Geometry check sheet. Reference: the model listing, model coordinates, mm. A direction names the side the tool comes from. Give positions to 0.01 mm unless a question says otherwise; leave off trailing zeros. Write each loop counter-clockwise with the first axis right and the second up, starting at its lowest first coordinate (ties: lowest second). Pieces come first, ordered by that corner, then holes.
(1) Depth check by flat-ended pin: P1, Ø12, axis at x = -33, z = 26.5, coming from the -Y side; P2, Ø4.5, axis at x = 50, y = -25, coming from the +Z side. Enter the tip coordinate at first touch or a pass-through.
(2) Cross-section at A-A (y = -31.5). Record the boundary of the cut face in (x, z).
(3) Thickness scan on line 1 along X through (y, z) = (-25, -96.25); line 2 along Z through (x, y) = (10, -27); line 3 along Y through (x, z) = (-50, -96). Record the ranges inside material, lowest first.
(4) Mould release check, pull along Z, two halves, no side actions. Record for faces 3 (the flat face through (-2, -22, -100)), 4 (the flat face through (-12, -45, -96)), 5 (the flat face through (-2, -30, 90)), 6 (the flat face through (-2, -15, 1)): +Z half, -Z half, draft (parallel to the pull), parting line (faces both ways), or undercut.
(5) Cross-section at B-B (x = -65). Record the boundary of the cut face in (y, z).
(6) Tool access check on faces 1 (the flat face through (-150, -22, -1)), 2 (the flat face through (-140, -30, -1)). Record the directions out of +Z, -Z, +X, -X, +Y, -Y that give a thin tool (end or side, any length) a straight path to the whole face; none if there is none.
(7) Cross-section at C-C (z = 74). Record the boundary of the cut face in (x, y), and give its area (3 significant figures).
```python
from build123d import *

# Parameters (mm, degrees)
F0_W     = 300
F0_H     = 200
F1_DEPTH = 45
F2_W     = 280
F2_H     = 180
F3_DEPTH = 30
F4_R     = 2.5
F5_DEPTH = 200.001


with BuildPart() as f1:
    # F0 (on Front) → F1 (new body)
    with BuildSketch(Plane.XZ):
        Rectangle(F0_W, F0_H)
    extrude(amount=F1_DEPTH)

    # F2 (on face) → F3 (cut)
    with BuildSketch(Plane.XZ.offset(45)):
        Rectangle(F2_W, F2_H)
    extrude(amount=-F3_DEPTH, mode=Mode.SUBTRACT)

    # F4 (on face) → F5 (cut, through all)
    with BuildSketch(Plane(origin=(0, 0, -100), x_dir=(1, 0, 0), z_dir=(0, 0, -1))):
        with Locations((-50, 25)):
            Circle(F4_R)
        with Locations((0, 25)):
            Circle(F4_R)
        with Locations((50, 25)):
            Circle(F4_R)
    extrude(amount=-F5_DEPTH, mode=Mode.SUBTRACT)


solid = f1.part
```
Reply:
1. P1: stops at y = -15
1. P2: passes through
2. outline: (-150, -100) - (150, -100) - (150, 100) - (-150, 100) - close; hole (-140, -90) - (140, -90) - (140, 90) - (-140, 90) - close
3. line 1: x = -150 to -52.5, -47.5 to -2.5, 2.5 to 47.5, 52.5 to 150
3. line 2: z = -100 to -90, 90 to 100
3. line 3: y = -45 to -27.5, -22.5 to 0
4. face 3: -Z half
4. face 4: draft
4. face 5: undercut
4. face 6: undercut
5. outline: (-45, -100) - (0, -100) - (0, 100) - (-45, 100) - (-45, 90) - (-15, 90) - (-15, -90) - (-45, -90) - close
6. face 1: +Z, -Z, -X, +Y, -Y
6. face 2: -Y
7. outline: (-150, -45) - (-140, -45) - (-140, -15) - (140, -15) - (140, -45) - (150, -45) - (150, 0) - (-150, 0) - close
7. area: 5,100 mm2
